Source: CAD feature listing. Evaluate the final solid. Frame: model axes, mm. A direction names the side the tool comes from. Coordinates: 2 decimals unless noted, no trailing zeros. Loops run counter-clockwise (first coordinate to the right, second up) from the corner with the lowest first, then second, coordinate; pieces in that order, holes last. Notation, with made-up numbers: (53, 79) -> (75, 79) arc R17 ccw to (75, 91) -> close; hole circle Ø4 at (77.5, 34). An arc over 180 degrees is marked (long way). Answer as CSV lines item,"result".
from build123d import *

# Parameters (mm, degrees)
SKETCH_2_W          = 19.6
SKETCH_2_H          = 40.4
EXTRUDE_2_DEPTH     = 35.9
SKETCH_8_W          = 19.6
SKETCH_8_H          = 36
EXTRUDE_4_DEPTH     = 2.5
EXTRUDE_5_DEPTH     = 7.3
EXTRUDE_6_DEPTH     = 7.3
EXTRUDE_7_DEPTH     = 7.3
SKETCH_13_R         = 6.4
EXTRUDE_8_DEPTH     = 2
SKETCH_15_R         = 2.9
EXTRUDE_9_DEPTH     = 3.5
SKETCH_16_W         = 19.6
SKETCH_16_H         = 9.65
EXTRUDE_10_DEPTH    = 0.01
SKETCH_17_R         = 1
CUT_EXTRUDE_1_DEPTH = 10
CUT_EXTRUDE_2_DEPTH = 10
SKETCH_19_R         = 1
CUT_EXTRUDE_3_DEPTH = 10


with BuildPart() as part:
    # ｽｹｯﾁ2 → ﾎﾞｽ - 押し出し2 (new body)
    with BuildSketch(Plane.XY):
        with Locations((25.664618486, 0.22320442)):
            Rectangle(SKETCH_2_W, SKETCH_2_H)
    extrude(amount=EXTRUDE_2_DEPTH)

    # ｽｹｯﾁ8 → ﾎﾞｽ - 押し出し4 (add)
    with BuildSketch(Plane.XY.offset(35.9)):
        with Locations((25.664618486, 2.42320442)):
            Rectangle(SKETCH_8_W, SKETCH_8_H)
    extrude(amount=EXTRUDE_4_DEPTH)

    # ｽｹｯﾁ9 → ﾎﾞｽ - 押し出し5 (add)
    with BuildSketch(Plane(origin=(0, 20.42320442, 0), x_dir=(1, 0, 0), z_dir=(0, 1, 0))):
        Polygon((35.464618486, -31.499834605), (35.464618486, -25.499834605), (25.664618486, -25.499834605), (15.864618486, -25.499834605), (15.864618486, -31.499834605), align=None)
    extrude(amount=EXTRUDE_5_DEPTH)

    # ｽｹｯﾁ10 → ﾎﾞｽ - 押し出し6 (add)
    with BuildSketch(Plane.XZ.offset(19.97679558)):
        Polygon((15.864618486, 31), (15.864618486, 25), (25.664618486, 25), (35.464618486, 25), (35.464618486, 31), align=None)
    extrude(amount=EXTRUDE_6_DEPTH)

    # ｽｹｯﾁ11 → ﾎﾞｽ - 押し出し7 (add)
    with BuildSketch(Plane(origin=(0, 20.42320442, 0), x_dir=(1, 0, 0), z_dir=(0, 1, 0))):
        Polygon((29.464618486, -3), (25.664618486, -3), (21.864618486, -3), (21.864618486, -6), (29.464618486, -6), align=None)
    extrude(amount=EXTRUDE_7_DEPTH)

    # ｽｹｯﾁ13 → ﾎﾞｽ - 押し出し8 (add)
    with BuildSketch(Plane.XY.offset(38.4)):
        with Locations((25.664618486, 10.62320442)):
            Circle(SKETCH_13_R)
    extrude(amount=EXTRUDE_8_DEPTH)

    # ｽｹｯﾁ15 → ﾎﾞｽ - 押し出し9 (add)
    with BuildSketch(Plane.XY.offset(40.4)):
        with Locations((25.664618486, 10.62320442)):
            Circle(SKETCH_15_R)
    extrude(amount=EXTRUDE_9_DEPTH)

    # ｽｹｯﾁ16 → ﾎﾞｽ - 押し出し10 (add)
    with BuildSketch(Plane.XY.offset(38.4)):
        with Locations((25.664618486, -6.75179558)):
            Rectangle(SKETCH_16_W, SKETCH_16_H)
    extrude(amount=EXTRUDE_10_DEPTH)

    # ｽｹｯﾁ17 → ｶｯﾄ - 押し出し1 (cut)
    with BuildSketch(Plane.XY.offset(31.499834605)):
        with Locations((31.064618486, 24.72320442)):
            Circle(SKETCH_17_R)
    extrude(amount=-CUT_EXTRUDE_1_DEPTH, mode=Mode.SUBTRACT)

    # ｽｹｯﾁ18 → ｶｯﾄ - 押し出し2 (cut)
    with BuildSketch(Plane.XY.offset(31.499834605)):
        with BuildLine():
            ThreePointArc((21.264618486, 24.72320442), (20.971725267, 25.430311201), (20.264618486, 25.72320442))
            Line((20.264618486, 25.72320442), (20.264618486, 24.72320442))
            Line((20.264618486, 24.72320442), (19.264618486, 24.72320442))
            ThreePointArc((19.264618486, 24.72320442), (20.264618486, 23.72320442), (21.264618486, 24.72320442))
        make_face()
        with BuildLine():
            Line((20.264618486, 24.72320442), (20.264618486, 25.72320442))
            ThreePointArc((20.264618486, 25.72320442), (19.557511705, 25.430311201), (19.264618486, 24.72320442))
            Line((19.264618486, 24.72320442), (20.264618486, 24.72320442))
        make_face()
    extrude(amount=-CUT_EXTRUDE_2_DEPTH, mode=Mode.SUBTRACT)

    # ｽｹｯﾁ19 → ｶｯﾄ - 押し出し3 (cut)
    with BuildSketch(Plane.XY.offset(31)):
        with Locations((20.264618486, -24.27679558)):
            Circle(SKETCH_19_R)
        with Locations((31.064618486, -24.27679558)):
            Circle(SKETCH_19_R)
    extrude(amount=-CUT_EXTRUDE_3_DEPTH, mode=Mode.SUBTRACT)


solid = part.part
(1) Pin query (flat end, axial travel): pin 1 Ø8 at (x, y) = (26.5, 25.5) entering from -Z; pin 2 Ø2 at (x, y) = (24.5, 25.5) entering from +Z; pin 3 Ø10 at (x, z) = (29.5, 17) entering from -Y. Return the tip coordinate at first contact, or that it passes through.
Computed values:
pin 1,"z = 3"
pin 2,"z = 31.5"
pin 3,"y = -19.98"
(2) Cut plane C-C (y = -4.5). Return the cut outline in (x, z), then the cut area to 3 significant figures.
Computed values:
outline,"(15.86, 0) -> (35.46, 0) -> (35.46, 38.41) -> (15.86, 38.41) -> close"
area,"753 mm^2"
(3) Cut plane B-B (z = 4.5). Return the cut outline in (x, y), then the cut area to 3 significant figures.
Computed values:
outline,"(15.86, -19.98) -> (35.46, -19.98) -> (35.46, 20.42) -> (29.46, 20.42) -> (29.46, 27.72) -> (21.86, 27.72) -> (21.86, 20.42) -> (15.86, 20.42) -> close"
area,"847 mm^2"
(4) Material intervals for L1, parallel to Z at x = 18, y = -21; L2, parallel to Z at x = 22.25, y = 12; L3, parallel to Y at x = 31.25, z = 20.5, sorted ascending. Write a range as [from, to].
Computed values:
L1,"[25, 31]"
L2,"[0, 40.4]"
L3,"[-19.98, 20.42]"
(5) Draft query along Y for faces 4 (the flat face through (26, 11, 43.9)), 5 (the cylindrical face through (30.271, 24.115, 28.542)), 6 (the flat face through (26, -15.577, 37)). Return one class per face: released by +Y, released by -Y, zero draft, split by the parting line, or undercut.
Computed values:
face 4,"zero draft"
face 5,"undercut"
face 6,"released by -Y"
(6) Access query for faces 1 (the flat face through (26, -19.977, 12)), 2 (the flat face through (21.865, 24, 4)), 3 (the cylindrical face through (31.577, 8.172, 39.386)). Directions: +Z, -Z, +X, -X, +Y, -Y. A direction counts if a zero-diameter tool reaches every point of the face in a straight line with its end or side. Return the directions, or none.
Computed values:
face 1,"-Z, +X, -X, -Y"
face 2,"-Z, -X, +Y"
face 3,"+Z"
(7) Cut plane A-A (x = 30.75). State how many separate pieces and enclosed holes the cut face has, then the cut area to 3 significant figures.
Computed values:
separate pieces,"3"
enclosed holes,"0"
area,"1,620 mm^2"
